from build123d import *

# Parameters (mm, degrees)
BOSS_EXTRUDE1_DEPTH = 25.4
CUT_EXTRUDE1_DEPTH  = 6.35
CUT_EXTRUDE2_DEPTH  = 6.35


with BuildPart() as part:
    # Sketch1 → Boss-Extrude1 (new body, symmetric)
    with BuildSketch(Plane.XY):
        Polygon((-31.75, 22.225), (-31.75, 12.7), (-17.4625, 12.7), (-17.4625, 9.525), (-11.1125, 9.525), (-11.1125, 12.7), (3.175, 12.7), (3.175, 0), (0, 0), (0, -6.35), (3.175, -6.35), (3.175, -12.7), (-11.1125, -12.7), (-11.1125, -9.525), (-17.4625, -9.525), (-17.4625, -12.7), (-31.75, -12.7), (-31.75, -22.225), (12.7, -22.225), (12.7, 22.225), align=None)
    extrude(amount=BOSS_EXTRUDE1_DEPTH, both=True)

    # Sketch2 → Cut-Extrude1 (cut)
    with BuildSketch(Plane.ZY.offset(17.4625)):
        with BuildLine():
            ThreePointArc((3.175, 12.7), (2.245064024, 10.454935963), (-1.9e-08, 9.525))
            Line((-1.9e-08, 9.525), (25.4, 9.525))
            Line((25.4, 9.525), (25.4, 12.7))
            Line((25.4, 12.7), (3.175, 12.7))
        make_face()
        with BuildLine():
            Line((-3.175, 12.7), (-25.4, 12.7))
            Line((-25.4, 12.7), (-25.4, 9.525))
            Line((-25.4, 9.525), (-1.9e-08, 9.525))
            ThreePointArc((-1.9e-08, 9.525), (-2.245064037, 10.454935976), (-3.175, 12.7))
        make_face()
        with BuildLine():
            Line((-2e-09, -9.525), (-25.4, -9.525))
            Line((-25.4, -9.525), (-25.4, -12.7))
            Line((-25.4, -12.7), (-3.175, -12.7))
            ThreePointArc((-3.175, -12.7), (-2.245064031, -10.454935971), (-2e-09, -9.525))
        make_face()
        with BuildLine():
            Line((25.4, -9.525), (-2e-09, -9.525))
            ThreePointArc((-2e-09, -9.525), (2.245064029, -10.454935969), (3.175, -12.7))
            Line((3.175, -12.7), (25.4, -12.7))
            Line((25.4, -12.7), (25.4, -9.525))
        make_face()
    extrude(amount=-CUT_EXTRUDE1_DEPTH, mode=Mode.SUBTRACT)

    # Sketch3 → Cut-Extrude2 (cut)
    with BuildSketch(Plane(origin=(0, 0, 0), x_dir=(1, 0, 0), z_dir=(0, 1, 0))):
        with BuildLine():
            Line((0, 0), (0, -25.4))
            Line((0, -25.4), (3.175, -25.4))
            Line((3.175, -25.4), (3.175, -3.175))
            ThreePointArc((3.175, -3.175), (0.92993597, -2.24506403), (0, 0))
        make_face()
    cut_extrude2 = extrude(amount=-CUT_EXTRUDE2_DEPTH, mode=Mode.SUBTRACT)

    # Mirror1: Cut-Extrude2 across plane
    add(cut_extrude2.mirror(Plane.XY), mode=Mode.SUBTRACT)


solid = part.part
Verification items for the finished model (mm, model axes). A direction names the side the tool comes from. Coordinates: 2 decimals unless noted, no trailing zeros. Write each loop counter-clockwise with the first axis right and the second up, starting at its lowest first coordinate (ties: lowest second). Pieces come first, ordered by that corner, then holes. Notation, with made-up numbers: (-17, 28) -> (34, 28) arc R20 cw to (34, 43) -> close; hole circle Ø4 at (-25, 23). An arc over 180 degrees is marked (long way). One line per item, written item: value. Start each with the question number.
Q1. Access from +Z, -Z, +X, -X, +Y, -Y to the whole of each face (thin tool, end or side, straight path). Record for faces 1 (the flat face through (5, 0, -25.4)), 2 (the flat face through (-11.112, -11, 0)), 3 (the flat face through (2, -6.35, 0)).
Q2. Cross-section at A-A on x = -14. Enter the section's corners in (y, z) (3 decimals), and give its area (3 significant figures).
Q3. Go/stop test with flat-tipped pins: P1, Ø1, axis at y = 12, z = 0, coming from the -X side; P2, Ø5, axis at x = -18.5, y = 6, coming from the +Z side; P3, Ø1.5, axis at y = -9.5, z = -11, coming from the -X side (3 decimals). Record where each tip stops, or that it passes through.
Q4. Mould release check, pull along X, two halves, no side actions. Record for faces 4 (the flat face through (-11.112, 11, 0)), 5 (the flat face through (12.7, 0, 0)), 6 (the flat face through (-9, 22.225, 0)), 7 (the flat face through (-17.462, 11, 0)): pulls with the +X half, pulls with the -X half, needs draft (parallel to the pull), parting line crosses it, or undercut.
Q5. Cross-section at B-B on z = -13.5. Enter the section's corners in (x, y) (3 decimals).
Q6. Cross-section at D-D on y = 1. Enter the section's corners in (x, z) (3 decimals).
Q7. Thickness scan on L1, parallel to Y at x = -14.5, z = 16 (3 decimals); L2, parallel to X at y = 12.5, z = 0 (1 decimal); L3, parallel to Y at x = -16.5, z = -1 (3 decimals). Record the ranges inside material, lowest first. Write a range as from..to.
Q8. Cross-section at C-C on x = -5. Enter the section's corners in (y, z) (3 decimals), and give its area (3 significant figures).
Checked values:
1. face 1: -Z, +X, -X, +Y, -Y
1. face 2: +Z, -Z
1. face 3: +Z, -Z, -X
2. outline: (-22.225, -25.4) -> (-12.7, -25.4) -> (-12.7, -3.175) arc R3.175 ccw to (-12.7, 3.175) -> (-12.7, 25.4) -> (-22.225, 25.4) -> close; (12.7, -25.4) -> (22.225, -25.4) -> (22.225, 25.4) -> (12.7, 25.4) -> (12.7, 3.175) arc R3.175 ccw to (12.7, -3.175) -> close
2. area: 999 mm²
3. P1: stops at x = -17.46
3. P2: passes through
3. P3: stops at x = 3.175
4. face 4: undercut
4. face 5: pulls with the +X half
4. face 6: needs draft
4. face 7: pulls with the -X half
5. outline: (-31.75, -22.225) -> (12.7, -22.225) -> (12.7, 22.225) -> (-31.75, 22.225) -> (-31.75, 12.7) -> (3.175, 12.7) -> (3.175, -12.7) -> (-31.75, -12.7) -> close
6. outline: (3.175, -25.4) -> (12.7, -25.4) -> (12.7, 25.4) -> (3.175, 25.4) -> close
7. L1: y = -22.225..-12.7, 12.7..22.225
7. L2: x = -17.5..-11.1, 3.2..12.7
7. L3: y = -22.225..-9.687, 9.687..22.225
8. outline: (-22.225, -25.4) -> (-12.7, -25.4) -> (-12.7, 25.4) -> (-22.225, 25.4) -> close; (12.7, -25.4) -> (22.225, -25.4) -> (22.225, 25.4) -> (12.7, 25.4) -> close
8. area: 968 mm²
